```python
from build123d import *

# Parameters (mm, degrees)
EXTRUDE_1_DEPTH     = 40
CHAMFER_1_SIZE      = 5
SKETCH_3_R          = 4.25
CUT_EXTRUDE_1_DEPTH = 67.520673478
SKETCH_4_R          = 4.25
CUT_EXTRUDE_2_DEPTH = 40


with BuildPart() as part:
    # 草图1 → 凸台-拉伸1 (new body)
    with BuildSketch(Plane.XY):
        Polygon((0, 0), (40, 0), (40, 40), (37.5, 40), (35, 35), (35, 26.322499125), (36.120266103, 25.614016347), (35, 24.905533569), (35, 19.233332915), (36.120266103, 18.524850137), (35, 17.816367359), (35, 5), (22.183632641, 5), (21.475149863, 3.879733897), (20.766667085, 5), (15.094466431, 5), (14.385983653, 3.879733897), (13.677500875, 5), (5, 5), (0, 2.5), align=None)
    extrude(amount=EXTRUDE_1_DEPTH)

    # 倒角1
    chamfer_1_edges = [part.edges().sort_by_distance(p)[0] for p in [
        (35, 5, 20),
    ]]
    chamfer(chamfer_1_edges, length=CHAMFER_1_SIZE)

    # 草图3 → 切除-拉伸1 (cut, through all)
    with BuildSketch(Plane(origin=(0, 5, 0), x_dir=(1, 0, 0), z_dir=(0, 1, 0))):
        with Locations(Location((15, -20, 0), (0, 0, 180))):
            Circle(SKETCH_3_R)
    extrude(amount=-CUT_EXTRUDE_1_DEPTH, mode=Mode.SUBTRACT)

    # 草图4 → 切除-拉伸2 (cut)
    with BuildSketch(Plane.ZY.offset(-35)):
        with Locations((20, 25)):
            Circle(SKETCH_4_R)
    extrude(amount=-CUT_EXTRUDE_2_DEPTH, mode=Mode.SUBTRACT)


solid = part.part
```
Build history of the part. All positions in model axes, mm. A direction names the side the tool comes from. Coordinates: 2 decimals unless noted, no trailing zeros. Order: outer loops, then holes, each group sorted by start corner. A loop starts at its lowest first (then second) coordinate and runs counter-clockwise, first axis right, second up. Notation, with made-up numbers: (-39, 57) -> (3, 57) arc R14 cw to (3, 74) -> close; hole circle Ø2 at (73, 46.5). An arc over 180 degrees is marked (long way). Answer in a Markdown table with one row per item. Add a question column.
Q1. Wall check: line 1 along Z through (x, y) = (36, 25); line 2 along Y through (x, z) = (38.3, 20); line 3 along X through (y, z) = (24.5, 10.5). Give the ranges that are in metal, low to high. Write a range as [from, to].
Q2. Band-saw the part on C-C, the plane z = 4. List the corners of the cut face in (x, y).
Q3. Band-saw the part on A-A, the plane y = 23. List the corners of the cut face in (x, z), then the cut area to 4 significant figures.
Q4. Drop flat-ended pins along their axis: pin 1 (8.5 mm diameter, centred on x = 24.5, z = 10, fed in from +Y); pin 2 (4.5 mm diameter, centred on y = 28.5, z = 12, fed in from -X); pin 3 (7.5 mm diameter, centred on x = 15, z = 20, fed in from +Y); pin 4 (6.5 mm diameter, centred on y = 13, z = 27, fed in from -X). Give the stop position or say it passes through.
Q5. Band-saw the part on B-B, the plane z = 20. List the corners of the cut face in (x, y).
Q6. Which spindle directions (+Z, -Z, +X, -X, +Y, -Y) get a long thin tool onto all of the face, cutting with end or side? Do faces 4 (the face through (33, 7, 0)), 5 (the face through (20, 5, 20)). Say none if no direction does.
Q7. Band-saw the part on D-D, the plane y = 15. List the corners of the cut face in (x, z).
Q8. Mould opens along X. For faces 1 (the face through (35, 31, 20)), 2 (the face through (21.126, 4.432, 19.72)), 3 (the face through (26, 5, 20)) say: +X half, -X half, draft (parallel to the pull), parting line (faces both ways), or undercut.
Answers follow:
| question | item | result |
|---|---|---|
| 1 | line 1 | [0, 15.75], [24.25, 40] |
| 1 | line 2 | [0, 20.75], [29.25, 40] |
| 1 | line 3 | [35, 40] |
| 2 | outline | (0, 0) -> (40, 0) -> (40, 40) -> (37.5, 40) -> (35, 35) -> (35, 26.32) -> (36.12, 25.61) -> (35, 24.91) -> (35, 19.23) -> (36.12, 18.52) -> (35, 17.82) -> (35, 10) -> (30, 5) -> (22.18, 5) -> (21.48, 3.88) -> (20.77, 5) -> (15.09, 5) -> (14.39, 3.88) -> (13.68, 5) -> (5, 5) -> (0, 2.5) -> close |
| 3 | outline | (35, 0) -> (40, 0) -> (40, 16.25) -> (35, 16.25) -> close; (35, 23.75) -> (40, 23.75) -> (40, 40) -> (35, 40) -> close |
| 3 | area | 162.5 mm^2 |
| 4 | pin 1 | y = 5 |
| 4 | pin 2 | x = 35 |
| 4 | pin 3 | through |
| 4 | pin 4 | x = 34.75 |
| 5 | outline | (0, 0) -> (10.75, 0) -> (10.75, 5) -> (5, 5) -> (0, 2.5) -> close; (19.25, 0) -> (40, 0) -> (40, 20.75) -> (35, 20.75) -> (35, 19.23) -> (36.12, 18.52) -> (35, 17.82) -> (35, 10) -> (30, 5) -> (22.18, 5) -> (21.48, 3.88) -> (20.77, 5) -> (19.25, 5) -> close; (35, 29.25) -> (40, 29.25) -> (40, 40) -> (37.5, 40) -> (35, 35) -> close |
| 6 | face 4 | -Z, +X, -X, +Y, -Y |
| 6 | face 5 | +Z, -Z, -X, +Y |
| 7 | outline | (35, 0) -> (40, 0) -> (40, 40) -> (35, 40) -> close |
| 8 | face 1 | -X half |
| 8 | face 2 | undercut |
| 8 | face 3 | draft |
